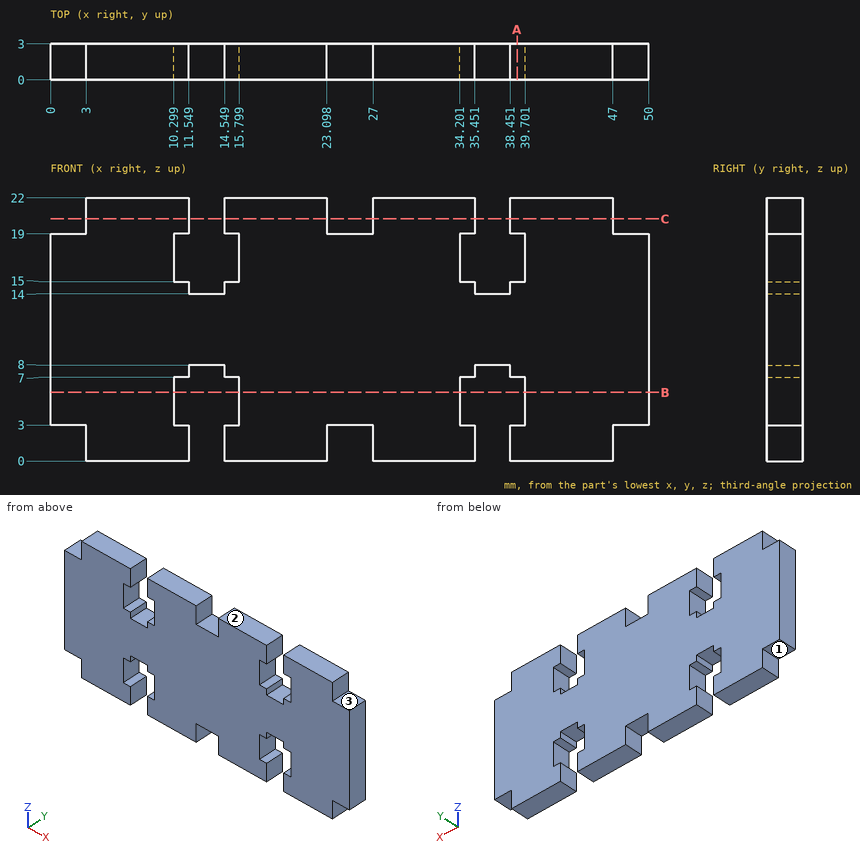
Here's the drawing with two shaded views (mm, measured from the low corner). I have some questions. A direction names the side the tool comes from. Coordinates: 2 decimals unless noted, no trailing zeros. Write each loop counter-clockwise with the first axis right and the second up, starting at its lowest first coordinate (ties: lowest second). Pieces come first, ordered by that corner, then holes.
Item 1: I want a section at C-C on z = 20.25. Write out the boundary of the cut face in (x, y).
Item 2: I want a section at B-B on z = 5.75. Write out the boundary of the cut face in (x, y).
Item 3: Will these pins go through, and if not, where does the flat tip stop? pin 1 (1.5 mm diameter, centred on y = 1.5, z = 1, fed in from -X); pin 2 (0.9 mm diameter, centred on x = 12.5, y = 2, fed in from -Z).
Item 4: If I drill on line 1 (X direction, y = 2.2, z = 16.75); line 2 (X direction, y = 2.65, z = 7.75); line 3 (Z direction, x = 11, y = 1.4), over which ranges is the centre line in solid material (lowest first)?
Item 5: I want a section at A-A on x = 39. Write out the boundary of the cut face in (y, z), and give its area (3 significant figures).
Item 6: On a 3-axis mill with a long thin cutter (end or side, diameter ignored), from which of +Z, -Z, +X, -X, +Y, -Y can I reach the whole of each face in a straight line? I mean the marked faces 1, 2 and 3. Say none if no direction works.
Findings below:
1. outline: (3, 0) - (11.55, 0) - (11.55, 3) - (3, 3) - close; (14.55, 0) - (23.1, 0) - (23.1, 3) - (14.55, 3) - close; (27, 0) - (35.45, 0) - (35.45, 3) - (27, 3) - close; (38.45, 0) - (47, 0) - (47, 3) - (38.45, 3) - close
2. outline: (0, 0) - (10.3, 0) - (10.3, 3) - (0, 3) - close; (15.8, 0) - (34.2, 0) - (34.2, 3) - (15.8, 3) - close; (39.7, 0) - (50, 0) - (50, 3) - (39.7, 3) - close
3. pin 1: stops at x = 3
3. pin 2: stops at z = 8
4. line 1: x = 0 to 10.3, 15.8 to 34.2, 39.7 to 50
4. line 2: x = 0 to 11.55, 14.55 to 35.45, 38.45 to 50
4. line 3: z = 0 to 3, 7 to 15, 19 to 22
5. outline: (0, 0) - (3, 0) - (3, 3) - (0, 3) - close; (0, 7) - (3, 7) - (3, 15) - (0, 15) - close; (0, 19) - (3, 19) - (3, 22) - (0, 22) - close
5. area: 42.0 mm2
6. face 1: -Z, -X, +Y, -Y
6. face 2: +Z, +X, -X, +Y, -Y
6. face 3: +Z, +X, +Y, -Y
